from build123d import *

# Parameters (mm, degrees)
ESBO_O1_R                       = 0.6
RESSALTO_EXTRUS_O1_DEPTH        = 0.5
ESBO_O3_W                       = 4
ESBO_O3_H                       = 5
RESSALTO_EXTRUS_O2_DEPTH        = 1.5
ESBO_O4_W                       = 1
ESBO_O4_H                       = 0.6
RESSALTO_EXTRUS_O3_DEPTH        = 1
CHANFRO1_SIZE                   = 0.8
PADR_O_LINEAR1_COUNT            = 4
PADR_O_LINEAR1_PITCH            = 1.25
CHANFRO1_OF_PADR_O_LINEAR1_SIZE = 0.8
ESPELHAR1_START                 = -1.1
ESPELHAR1_DEPTH                 = 0.6
ESPELHAR1_START_2               = 0.15
ESPELHAR1_2_DEPTH               = 0.6
ESPELHAR1_START_3               = 1.4
ESPELHAR1_3_DEPTH               = 0.6
ESPELHAR1_START_4               = 2.65
ESPELHAR1_4_DEPTH               = 0.6
CHANFRO2_SIZE                   = 0.2


# Read off the part's stored shape, not the designer's step: Espelhar1
with BuildPart() as part:
    # Esboço1 → Ressalto-extrusão1 (new body)
    with BuildSketch(Plane.XY):
        with BuildLine():
            Line((-7, 9.2), (-5.5, 9.2))
            Line((-5.5, 9.2), (-5.5, 9.19))
            ThreePointArc((-5.5, 9.19), (-5.268614357, 8.631385643), (-4.71, 8.4))
            Line((-4.71, 8.4), (4.71, 8.4))
            ThreePointArc((4.71, 8.4), (5.268614357, 8.631385643), (5.5, 9.19))
            Line((5.5, 9.19), (5.5, 9.2))
            Line((5.5, 9.2), (7, 9.2))
            Line((7, 9.2), (7.5, 8.7))
            Line((7.5, 8.7), (7.5, 6.7))
            Line((7.5, 6.7), (7, 6.2))
            Line((7, 6.2), (6.5, 6.2))
            ThreePointArc((6.5, 6.2), (5.792893219, 5.907106781), (5.5, 5.2))
            Line((5.5, 5.2), (5.5, -5.2))
            ThreePointArc((5.5, -5.2), (5.792893219, -5.907106781), (6.5, -6.2))
            Line((6.5, -6.2), (7, -6.2))
            Line((7, -6.2), (7.5, -6.7))
            Line((7.5, -6.7), (7.5, -8.7))
            Line((7.5, -8.7), (7, -9.2))
            Line((7, -9.2), (5.5, -9.2))
            Line((5.5, -9.2), (5.5, -9.19))
            ThreePointArc((5.5, -9.19), (5.327193001, -8.772806999), (4.91, -8.6))
            Line((4.91, -8.6), (-4.91, -8.6))
            ThreePointArc((-4.91, -8.6), (-5.327193001, -8.772806999), (-5.5, -9.19))
            Line((-5.5, -9.19), (-5.5, -9.2))
            Line((-5.5, -9.2), (-7, -9.2))
            Line((-7, -9.2), (-7.5, -8.7))
            Line((-7.5, -8.7), (-7.5, -6.7))
            Line((-7.5, -6.7), (-7, -6.2))
            Line((-7, -6.2), (-6.5, -6.2))
            ThreePointArc((-6.5, -6.2), (-5.792893219, -5.907106781), (-5.5, -5.2))
            Line((-5.5, -5.2), (-5.5, 5.2))
            ThreePointArc((-5.5, 5.2), (-5.792893219, 5.907106781), (-6.5, 6.2))
            Line((-6.5, 6.2), (-7, 6.2))
            Line((-7, 6.2), (-7.5, 6.7))
            Line((-7.5, 6.7), (-7.5, 8.7))
            Line((-7.5, 8.7), (-7, 9.2))
        make_face()
        with Locations((-5.93, 7.7)):
            Circle(ESBO_O1_R, mode=Mode.SUBTRACT)
        with Locations(Location((5.93, 7.7, 0), (0, 0, 180))):
            Circle(ESBO_O1_R, mode=Mode.SUBTRACT)
        with Locations(Location((-5.93, -7.7, 0), (0, 0, 180))):
            Circle(ESBO_O1_R, mode=Mode.SUBTRACT)
        with Locations((5.93, -7.7)):
            Circle(ESBO_O1_R, mode=Mode.SUBTRACT)
    extrude(amount=RESSALTO_EXTRUS_O1_DEPTH)

    # Esboço3 → Ressalto-extrusão2 (add)
    with BuildSketch(Plane(origin=(0, 0, 0), x_dir=(-1, 0, 0), z_dir=(0, 0, -1))):
        with Locations((-0.5, 1.05)):
            Rectangle(ESBO_O3_W, ESBO_O3_H)
    extrude(amount=RESSALTO_EXTRUS_O2_DEPTH)

    # Esboço4 → Ressalto-extrusão3 (add)
    with BuildSketch(Plane(origin=(0, 0, 0), x_dir=(-1, 0, 0), z_dir=(0, 0, -1))):
        with Locations((2, 2.95)):
            Rectangle(ESBO_O4_W, ESBO_O4_H)
    ressalto_extrus_o3 = extrude(amount=RESSALTO_EXTRUS_O3_DEPTH)

    # Chanfro1
    chanfro1_edges = [part.edges().sort_by_distance(p)[0] for p in [
        (-2.5, 2.95, -1),
    ]]
    chamfer(chanfro1_edges, length=CHANFRO1_SIZE)

    # Padrão linear1: Ressalto-extrusão3 ×4
    with Locations(*[(0, -i * PADR_O_LINEAR1_PITCH, 0) for i in range(1, PADR_O_LINEAR1_COUNT)]):
        add(ressalto_extrus_o3)

    # Chanfro1 of Padrão linear1
    chanfro1_of_padr_o_linear1_edges = [part.edges().sort_by_distance(p)[0] for p in [
        (-2.5, 1.7, -1),
        (-2.5, 0.45, -1),
        (-2.5, -0.8, -1),
    ]]
    chamfer(chanfro1_of_padr_o_linear1_edges, length=CHANFRO1_OF_PADR_O_LINEAR1_SIZE)

    # Espelhar1 outline → Espelhar1 (add)
    with BuildSketch(Plane(origin=(0, 0, 0), x_dir=(1, 0, 0), z_dir=(0, 1, 0)).offset(ESPELHAR1_START)):
        Polygon((3.5, 0.2), (2.7, 1), (2.5, 1), (2.5, 0), (3.5, 0), align=None)
    extrude(amount=ESPELHAR1_DEPTH)

    # Espelhar1 2 outline → Espelhar1 2 (add)
    with BuildSketch(Plane(origin=(0, 0, 0), x_dir=(1, 0, 0), z_dir=(0, 1, 0)).offset(ESPELHAR1_START_2)):
        Polygon((3.5, 0.2), (2.7, 1), (2.5, 1), (2.5, 0), (3.5, 0), align=None)
    extrude(amount=ESPELHAR1_2_DEPTH)

    # Espelhar1 3 outline → Espelhar1 3 (add)
    with BuildSketch(Plane(origin=(0, 0, 0), x_dir=(1, 0, 0), z_dir=(0, 1, 0)).offset(ESPELHAR1_START_3)):
        Polygon((3.5, 0.2), (2.7, 1), (2.5, 1), (2.5, 0), (3.5, 0), align=None)
    extrude(amount=ESPELHAR1_3_DEPTH)

    # Espelhar1 4 outline → Espelhar1 4 (add)
    with BuildSketch(Plane(origin=(0, 0, 0), x_dir=(1, 0, 0), z_dir=(0, 1, 0)).offset(ESPELHAR1_START_4)):
        Polygon((3.5, 0.2), (2.7, 1), (2.5, 1), (2.5, 0), (3.5, 0), align=None)
    extrude(amount=ESPELHAR1_4_DEPTH)

    # Chanfro2
    chanfro2_edges = [part.edges().sort_by_distance(p)[0] for p in [
        (2.5, 1.05, -1.5),
        (0.5, -1.45, -1.5),
        (-1.5, 1.05, -1.5),
        (0.5, 3.55, -1.5),
    ]]
    chamfer(chanfro2_edges, length=CHANFRO2_SIZE)


solid = part.part
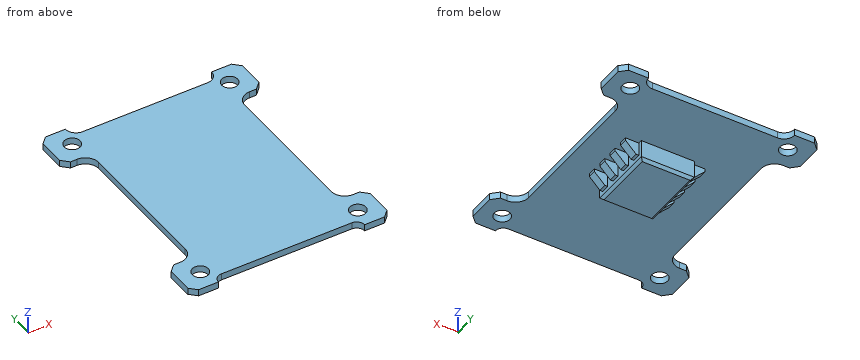
Verification items for the finished model (mm, model axes). Round coordinates to 2 decimals unless told otherwise and drop trailing zeros. Write each loop counter-clockwise with the first axis right and the second up, starting at its lowest first coordinate (ties: lowest second). Pieces come first, ordered by that corner, then holes.
(1) Section check D-D (y = -5). Enter the section's corners in (x, z).
Returned:
outline: (-5.5, 0) - (5.5, 0) - (5.5, 0.5) - (-5.5, 0.5) - close
(2) Section check B-B (x = -5.93). Enter the section's corners in (y, z).
Returned:
outline: (-9.2, 0) - (-8.3, 0) - (-8.3, 0.5) - (-9.2, 0.5) - close; (-7.1, 0) - (-6.02, 0) - (-6.02, 0.5) - (-7.1, 0.5) - close; (6.02, 0) - (7.1, 0) - (7.1, 0.5) - (6.02, 0.5) - close; (8.3, 0) - (9.2, 0) - (9.2, 0.5) - (8.3, 0.5) - close
(3) Material ranges on line 1 (Y direction, x = -5.93, z = 0.4); line 2 (Z direction, x = 4.5, y = -7); line 3 (Y direction, x = 0.5, z = 0.3), recorded low to high.
Returned:
line 1: y = -9.2 to -8.3, -7.1 to -6.02, 6.02 to 7.1, 8.3 to 9.2
line 2: z = 0 to 0.5
line 3: y = -8.6 to 8.4
(4) Section check A-A (y = 7.7). Enter the section's corners in (x, z).
Returned:
outline: (-7.5, 0) - (-6.53, 0) - (-6.53, 0.5) - (-7.5, 0.5) - close; (-5.33, 0) - (5.33, 0) - (5.33, 0.5) - (-5.33, 0.5) - close; (6.53, 0) - (7.5, 0) - (7.5, 0.5) - (6.53, 0.5) - close
(5) Section check C-C (x = 0). Enter the section's corners in (y, z), plus the area to 3 significant figures.
Returned:
outline: (-8.6, 0) - (-1.45, 0) - (-1.45, -1.3) - (-1.25, -1.5) - (3.35, -1.5) - (3.55, -1.3) - (3.55, 0) - (8.4, 0) - (8.4, 0.5) - (-8.6, 0.5) - close
area: 16.0 mm2
(6) Depth check by flat-ended pin: pin 1 Ø1 at (y, z) = (0, -1) entering from -X; pin 2 Ø0.5 at (x, z) = (3, -0.5) entering from -Y; pin 3 Ø1 at (y, z) = (4, 0) entering from +X. Enter the tip coordinate at first touch or a pass-through.
Returned:
pin 1: stops at x = -2.18
pin 2: stops at y = -1.1
pin 3: stops at x = 5.5
